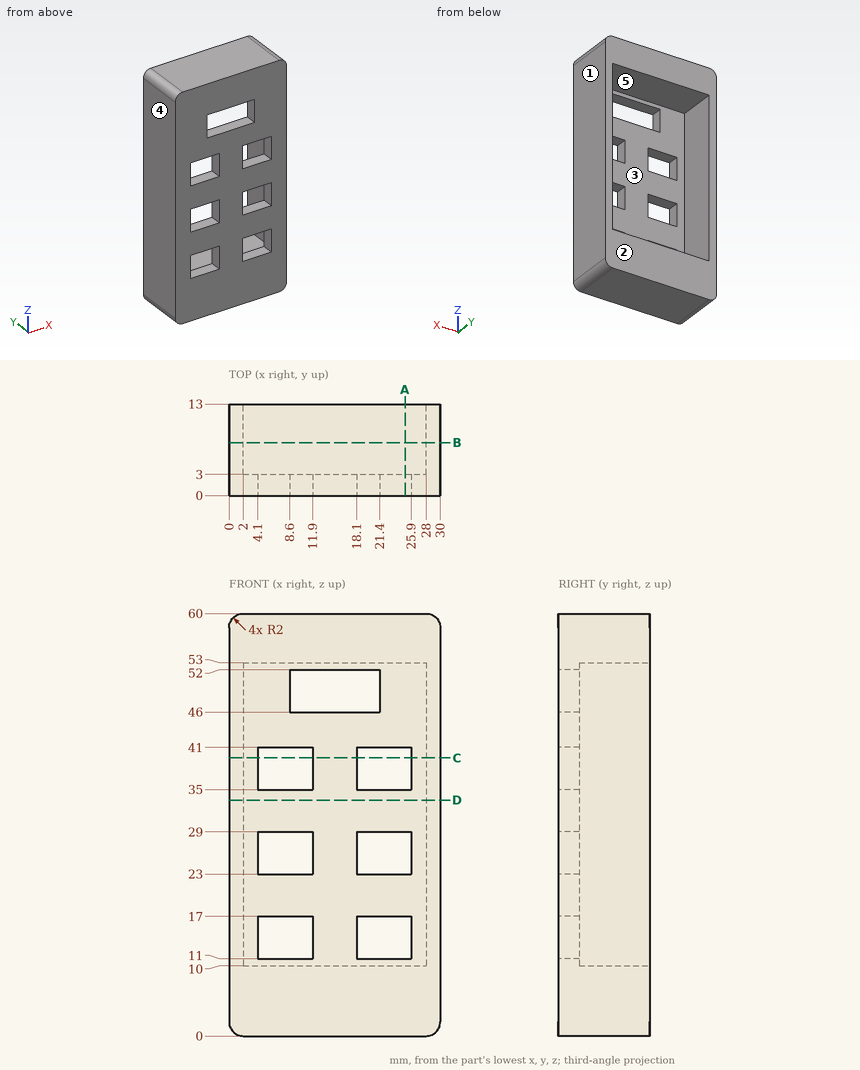
Design review of the part shown in the three views and the two pictorial views. Dimensions are in mm from the part's minimum x, y and z. A direction names the side the tool comes from. Round coordinates to 2 decimals unless told otherwise and drop trailing zeros. Loops run counter-clockwise (first coordinate to the right, second up) from the corner with the lowest first, then second, coordinate; pieces in that order, holes last. Notation, with made-up numbers: (86, 14.5) -> (138, 14.5) arc R7 cw to (138, 24.5) -> close; hole circle Ø11 at (-14, 26). An arc over 180 degrees is marked (long way). Answer as a JSON object with one key per item and string values. Group by question number.
1) We need section B-B on y = 7.5. Write out the cut boundary in (x, z).
2) We need section D-D on z = 33.5. Write out the cut boundary in (x, y), then the cut area to 3 significant figures.
3) For the marked faces 4 and 5, list the 3-axis set-ups (+Z, -Z, +X, -X, +Y, -Y) from which the entire face can be reached by the end or side of a thin tool; tool diameter is ignored.
4) We need section A-A on x = 25. Write out the cut boundary in (y, z).
5) Mouldability with a two-part tool opening along X and no side actions: class the marked faces 1, 2 and 3 as released by +X, released by -X, zero draft, split by the parting line, or undercut.
6) For line 1 (X direction, y = 3.75, z = 47); line 2 (Z direction, x = 24.5, y = 6.25); line 3 (X direction, y = 0.5, z = 25), list the stretches that pass through material, from the lowest coordinate up. Write a range as [from, to].
7) We need section C-C on z = 39.5. Write out the cut boundary in (x, y), then the cut area to 3 significant figures.
8) For pin 1 Ø10 at (x, z) = (18.5, 20.5) entering from +Y, flat-tipped, find the tip position at first contact; note if it passes through.
Result set:
{
 "1": {"outline": "(0, 2) arc R2 ccw to (2, 0) -> (28, 0) arc R2 ccw to (30, 2) -> (30, 58) arc R2 ccw to (28, 60) -> (2, 60) arc R2 ccw to (0, 58) -> close; hole (2, 10) -> (28, 10) -> (28, 53) -> (2, 53) -> close"},
 "2": {"outline": "(0, 0) -> (30, 0) -> (30, 13) -> (28, 13) -> (28, 3) -> (2, 3) -> (2, 13) -> (0, 13) -> close", "area": "130 mm²"},
 "3": {"face 4": "+Z, -Z, -X, +Y, -Y", "face 5": "+Y"},
 "4": {"outline": "(0, 0) -> (13, 0) -> (13, 10) -> (3, 10) -> (3, 11) -> (0, 11) -> close; (0, 17) -> (3, 17) -> (3, 23) -> (0, 23) -> close; (0, 29) -> (3, 29) -> (3, 35) -> (0, 35) -> close; (0, 41) -> (3, 41) -> (3, 53) -> (13, 53) -> (13, 60) -> (0, 60) -> close"},
 "5": {"face 1": "released by +X", "face 2": "zero draft", "face 3": "undercut"},
 "6": {"line 1": "[0, 2], [28, 30]", "line 2": "[0, 10], [53, 60]", "line 3": "[0, 4.1], [11.9, 18.1], [25.9, 30]"},
 "7": {"outline": "(0, 0) -> (4.1, 0) -> (4.1, 3) -> (2, 3) -> (2, 13) -> (0, 13) -> close; (11.9, 0) -> (18.1, 0) -> (18.1, 3) -> (11.9, 3) -> close; (25.9, 0) -> (30, 0) -> (30, 13) -> (28, 13) -> (28, 3) -> (25.9, 3) -> close", "area": "83.2 mm²"},
 "8": {"pin 1": "y = 3"}
}
